Geometry: final body of the model. Coordinates: model frame, mm. A direction names the side the tool comes from. Coordinates: 2 decimals unless noted, no trailing zeros. Order: outer loops, then holes, each group sorted by start corner. A loop starts at its lowest first (then second) coordinate and runs counter-clockwise, first axis right, second up. Notation, with made-up numbers: (-24, 89) - (13, 89) arc R14 ccw to (13, 116) - close; hole circle Ø4 at (50.5, -7.75). An arc over 180 degrees is marked (long way). Use a Markdown table: item, result. Add a question column.
```python
from build123d import *

# Parameters (mm, degrees)
AUFSATZ_LINEAR_AUSTRAGEN1_DEPTH  = 136
AUFSATZ_LINEAR_AUSTRAGEN2_DEPTH  = 2
AUFSATZ_LINEAR_AUSTRAGEN3_DEPTH  = 7
AUFSATZ_LINEAR_AUSTRAGEN6_DEPTH  = 2
LINEARES_MUSTER3_COUNT           = 2
LINEARES_MUSTER3_PITCH           = 12
SKIZZE12_W                       = 32
SKIZZE12_H                       = 14
SKIZZE12_R                       = 1.6
AUFSATZ_LINEAR_AUSTRAGEN14_DEPTH = 2
AUFSATZ_LINEAR_AUSTRAGEN15_DEPTH = 1
SCHNITT_LINEAR_START             = -2
SKIZZE14_R                       = 2.5
SCHNITT_LINEAR_AUSTRAGEN1_DEPTH  = 2


with BuildPart() as part:
    # Skizze1 → Aufsatz-Linear austragen1 (new body)
    with BuildSketch(Plane.XY):
        with BuildLine():
            Line((7.25, 0), (10.969655115, 0))
            Line((10.969655115, 0), (5.484827557, -9.5))
            Line((5.484827557, -9.5), (-5.484827557, -9.5))
            Line((-5.484827557, -9.5), (-10.969655115, 0))
            Line((-10.969655115, 0), (-7.25, 0))
            ThreePointArc((-7.25, 0), (0, -7.25), (7.25, 0))
        make_face()
    extrude(amount=AUFSATZ_LINEAR_AUSTRAGEN1_DEPTH)

    # Skizze2 → Aufsatz-Linear austragen2 (add)
    with BuildSketch(Plane.XY):
        with BuildLine():
            Line((7.25, 0), (-7.25, 0))
            ThreePointArc((-7.25, 0), (0, -7.25), (7.25, 0))
        make_face()
    extrude(amount=AUFSATZ_LINEAR_AUSTRAGEN2_DEPTH)

    # Skizze3 → Aufsatz-Linear austragen3 (add)
    with BuildSketch(Plane.XY.offset(133)):
        with BuildLine():
            Line((-8.3, 0), (-13.279056191, 0))
            Line((-13.279056191, 0), (-6.639528096, -11.5))
            Line((-6.639528096, -11.5), (6.639528096, -11.5))
            Line((6.639528096, -11.5), (13.279056191, 0))
            Line((13.279056191, 0), (8.3, 0))
            ThreePointArc((8.3, 0), (0, -8.3), (-8.3, 0))
        make_face()
    extrude(amount=AUFSATZ_LINEAR_AUSTRAGEN3_DEPTH)

    # Skizze7 → Aufsatz-Linear austragen6 (add)
    with BuildSketch(Plane.XY):
        Polygon((10.969655115, 0), (5.484827557, -9.5), (16, -9.5), align=None)
        Polygon((-5.484827557, -9.5), (-10.969655115, 0), (-16, -9.5), align=None)
    aufsatz_linear_austragen6 = extrude(amount=AUFSATZ_LINEAR_AUSTRAGEN6_DEPTH)

    # Lineares Muster3: Aufsatz-Linear austragen6 ×2
    with Locations(*[(0, 0, i * LINEARES_MUSTER3_PITCH) for i in range(1, LINEARES_MUSTER3_COUNT)]):
        add(aufsatz_linear_austragen6)

    # Skizze12 → Aufsatz-Linear austragen14 (add)
    with BuildSketch(Plane.XZ.offset(9.5)):
        with Locations((0, 7)):
            Rectangle(SKIZZE12_W, SKIZZE12_H)
        with Locations((-13, 7)):
            Circle(SKIZZE12_R, mode=Mode.SUBTRACT)
        with Locations((13, 7)):
            Circle(SKIZZE12_R, mode=Mode.SUBTRACT)
    extrude(amount=AUFSATZ_LINEAR_AUSTRAGEN14_DEPTH)

    # Skizze13 → Aufsatz-Linear austragen15 (add)
    with BuildSketch(Plane(origin=(0, 0, 0), x_dir=(1, 0, 0), z_dir=(0, 1, 0))):
        Polygon((8.3, -140), (10.789528096, -140), (10.789528096, -134.5), (9.169655115, -134.5), (9.169655115, -1), (-9.169655115, -1), (-9.169655115, -134.5), (-10.789528096, -134.5), (-10.789528096, -140), (-8.3, -140), (-8.3, -136), (-7.25, -136), (-7.25, -2), (7.25, -2), (7.25, -136), (8.3, -136), align=None)
    extrude(amount=AUFSATZ_LINEAR_AUSTRAGEN15_DEPTH)

    # Skizze14 → Schnitt-Linear austragen1 (cut)
    with BuildSketch(Plane(origin=(0, 0, 0), x_dir=(-1, 0, 0), z_dir=(0, 0, -1)).offset(SCHNITT_LINEAR_START)):
        Circle(SKIZZE14_R)
    extrude(amount=SCHNITT_LINEAR_AUSTRAGEN1_DEPTH, mode=Mode.SUBTRACT)


solid = part.part
```
1) Ray query, line 1 along Z through (x, y) = (9.5, -2.75); line 2 along Z through (x, y) = (13, -10); line 3 along Z through (x, y) = (6, -0.5). Return the intervals inside material, ascending.
2) Section A-A (z = 7). Return loops of the section in (x, y).
3) Section B-B (x = 0). Return loops of the section in (y, z), then the cut area to 3 significant figures.
4) Set-up query: faces 1 (the face through (0.18, -8.3, 137.97)), 2 (the face through (-8.2, -4.8, 6.9)), 3 (the face through (9.913, -5.83, 136.451)), 4 (the face through (-8.2, -4.8, 72.7)), 5 (the face through (11, -9.5, 7)). Return all of +Z, -Z, +X, -X, +Y, -Y with unobstructed straight access to the full face (end or side cutting, diameter ignored); none if empty.
5) Section C-C (z = 81). Return loops of the section in (x, y), then the cut area to 3 significant figures.
6) Draft query along Z for faces 6 (the face through (-13.45, -4.68, 12.99)), 7 (the face through (0, -9.5, 73)), 8 (the face through (0, -6, 0)). Return one class per face: pulls with the +Z half, pulls with the -Z half, needs draft (parallel to the pull), parting line crosses it, or undercut.
7) Pin query (flat end, axial travel): pin 1 (6 mm diameter, centred on y = -4.5, z = 23, fed in from +X); pin 2 (12 mm diameter, centred on x = -6, z = 85.5, fed in from -Y); pin 3 (0.8 mm diameter, centred on y = 0.5, z = 64, fed in from +X). Return the tip coordinate at first contact, or that it passes through.
Values follow:
| question | item | result |
|---|---|---|
| 1 | line 1 | z = 0 to 2, 12 to 14, 133 to 140 |
| 1 | line 2 | z = 0 to 5.4, 8.6 to 14 |
| 1 | line 3 | z = 0 to 2 |
| 2 | outline | (-16, -11.5) - (-14.6, -11.5) - (-14.6, -9.5) - (-16, -9.5) - close; (-11.4, -11.5) - (11.4, -11.5) - (11.4, -9.5) - (5.48, -9.5) - (10.97, 0) - (9.17, 0) - (9.17, 1) - (7.25, 1) - (7.25, 0) arc R7.25 cw to (-7.25, 0) - (-7.25, 1) - (-9.17, 1) - (-9.17, 0) - (-10.97, 0) - (-5.48, -9.5) - (-11.4, -9.5) - close; (14.6, -11.5) - (16, -11.5) - (16, -9.5) - (14.6, -9.5) - close |
| 3 | outline | (-11.5, 0) - (-2.5, 0) - (-2.5, 2) - (-7.25, 2) - (-7.25, 136) - (-8.3, 136) - (-8.3, 140) - (-11.5, 140) - (-11.5, 133) - (-9.5, 133) - (-9.5, 14) - (-11.5, 14) - close |
| 3 | area | 362 mm² |
| 4 | face 1 | +Z, +Y |
| 4 | face 2 | -X |
| 4 | face 3 | +Z, +X, -Y |
| 4 | face 4 | -X, -Y |
| 4 | face 5 | +X |
| 5 | outline | (-10.97, 0) - (-5.48, -9.5) - (5.48, -9.5) - (10.97, 0) - (9.17, 0) - (9.17, 1) - (7.25, 1) - (7.25, 0) arc R7.25 cw to (-7.25, 0) - (-7.25, 1) - (-9.17, 1) - (-9.17, 0) - close |
| 5 | area | 77.6 mm² |
| 6 | face 6 | needs draft |
| 6 | face 7 | undercut |
| 6 | face 8 | pulls with the -Z half |
| 7 | pin 1 | stops at x = 10.1 |
| 7 | pin 2 | stops at y = -9.5 |
| 7 | pin 3 | stops at x = 9.17 |
